```python
from build123d import *

# Parameters (mm, degrees)
F0_R     = 44.5718296496
F1_DEPTH = 59.713
F2_DEPTH = 25
F3_W     = 50.5398474634
F3_H     = 39.9477705359
F4_DEPTH = 128.1019449234
F5_SIZE  = 7


with BuildPart() as f1:
    # F0 (on Right) → F1 (new body)
    with BuildSketch(Plane.YZ):
        Circle(F0_R)
    extrude(amount=F1_DEPTH)

    # F2 (add): a face of the model
    f2_faces = [f1.faces().sort_by_distance(p)[0] for p in [
        (59.713, 0, 0),
    ]]
    extrude(f2_faces, amount=F2_DEPTH)

    # F3 (on face) → F4 (cut)
    with BuildSketch(Plane.YZ.offset(84.713)):
        with Locations((-2.7490835637, -1.037882641)):
            Rectangle(F3_W, F3_H)
    extrude(amount=-F4_DEPTH, mode=Mode.SUBTRACT)

    # F5
    f5_edges = [f1.edges().sort_by_distance(p)[0] for p in [
        (84.713, -44.57183, 0),
    ]]
    chamfer(f5_edges, length=F5_SIZE)


solid = f1.part
```
The listing builds one solid part. Answer for the finished solid, in the listing's coordinates (mm). A direction names the side the tool comes from. Round coordinates to 2 decimals unless told otherwise and drop trailing zeros. Loops run counter-clockwise (first coordinate to the right, second up) from the corner with the lowest first, then second, coordinate; pieces in that order, holes last. Notation, with made-up numbers: (71, -7) -> (116, -7) arc R24 cw to (116, 32) -> close; hole circle Ø7 at (-15, 77). An arc over 180 degrees is marked (long way). Use one line per item in the form item = value.
1. Find the intervals of material crossed by probe 1 along Z at (x, y) = (47, 8.5); probe 2 along Z at (x, y) = (28.5, 7); probe 3 along Y at (x, z) = (59, 3.5), in increasing order. Write a range as [from, to].
Answer key:
probe_1 = [-43.75, -21.01], [18.94, 43.75]
probe_2 = [-44.02, -21.01], [18.94, 44.02]
probe_3 = [-44.43, -28.02], [22.52, 44.43]
2. The part is cut by section A-A on z = 0. Determine the outline of the cut face in (x, y).
Answer key:
outline = (0, -44.57) -> (77.71, -44.57) -> (84.71, -37.57) -> (84.71, -28.02) -> (0, -28.02) -> close; (0, 22.52) -> (84.71, 22.52) -> (84.71, 37.57) -> (77.71, 44.57) -> (0, 44.57) -> close
3. Flat-ended cylindrical pins translate along their axes: pin 1 Ø10 at (x, y) = (34, 30) entering from +Z; pin 2 Ø4 at (x, y) = (26.5, 4.5) entering from -Z; pin 3 Ø5 at (x, z) = (44, 12) entering from -Y. Find the tip coordinate at first contact, or state that the pin passes through.
Answer key:
pin_1 = 36.9
pin_2 = -44.5
pin_3 = -43.55
4. The part is cut by section C-C on x = 15.5. Determine the outline of the cut face in (y, z), and give its area (3 significant figures).
Answer key:
outline = circle Ø89.14 at (0, 0); hole (-28.02, -21.01) -> (22.52, -21.01) -> (22.52, 18.94) -> (-28.02, 18.94) -> close
area = 4,220 mm²
5. For a pull along Z with two mould halves and no side action, classify faces 3 (the cylindrical face through (38.313, 23.962, 37.583)), 4 (the flat face through (43, -3, -21.012)), 5 (the flat face through (0, -1, 20)) as released by +Z, released by -Z, zero draft, split by the parting line, or undercut.
Answer key:
face_3 = split by the parting line
face_4 = undercut
face_5 = zero draft
6. The part is cut by section B-B on y = 0. Determine the outline of the cut face in (x, z), and give its area (3 significant figures).
Answer key:
outline = (0, -44.57) -> (77.71, -44.57) -> (84.71, -37.57) -> (84.71, -21.01) -> (0, -21.01) -> close; (0, 18.94) -> (84.71, 18.94) -> (84.71, 37.57) -> (77.71, 44.57) -> (0, 44.57) -> close
area = 4,120 mm²
7. A tool of negligible diameter and unlimited length cuts with its end or side. For faces 1 (the flat face through (84.713, 25, 1)), 2 (the flat face through (43, -28.019, -1)), from which of +Z, -Z, +X, -X, +Y, -Y can it reach the whole face along a straight path? Write none if from no direction.
Answer key:
face_1 = +Z, -Z, +X, +Y, -Y
face_2 = +X, -X
